from build123d import *

# Parameters (mm, degrees)
SKETCH_1_R      = 18
SKETCH_1_R_2    = 12
SKETCH_1_R_3    = 1.25
EXTRUDE_1_DEPTH = 5
EXTRUDE_START   = -2
SKETCH_2_R      = 12
SKETCH_2_R_2    = 10
EXTRUDE_2_DEPTH = 2
FILLET_1_R      = 1


with BuildPart() as part:
    # 草图1 → 凸台-拉伸1 (new body)
    with BuildSketch(Plane.XY):
        Circle(SKETCH_1_R)
        Circle(SKETCH_1_R_2, mode=Mode.SUBTRACT)
        with Locations((0, 15)):
            Circle(SKETCH_1_R_3, mode=Mode.SUBTRACT)
        with Locations((-15, 0)):
            Circle(SKETCH_1_R_3, mode=Mode.SUBTRACT)
        with Locations((0, -15)):
            Circle(SKETCH_1_R_3, mode=Mode.SUBTRACT)
        with Locations((15, 0)):
            Circle(SKETCH_1_R_3, mode=Mode.SUBTRACT)
    extrude(amount=EXTRUDE_1_DEPTH)

    # 草图2 → 凸台-拉伸2 (add)
    with BuildSketch(Plane.XY.offset(5).offset(EXTRUDE_START)):
        Circle(SKETCH_2_R)
        Circle(SKETCH_2_R_2, mode=Mode.SUBTRACT)
    extrude(amount=EXTRUDE_2_DEPTH)

    # 圆角1
    fillet_1_edges = [part.edges().sort_by_distance(p)[0] for p in [
        (-18, 0, 5),
    ]]
    fillet(fillet_1_edges, radius=FILLET_1_R)


solid = part.part
Geometry check sheet. Reference: the model listing, model coordinates, mm. A direction names the side the tool comes from. Round coordinates to 2 decimals unless told otherwise and drop trailing zeros. Order: outer loops, then holes, each group sorted by start corner. A loop starts at its lowest first (then second) coordinate and runs counter-clockwise, first axis right, second up. Notation, with made-up numbers: M -15.5,18.5 L 30.5,18.5 A18 ccw 30.5,42.5 Z; hole C -30,-35 d9. An arc over 180 degrees is marked long. Answer in a Markdown table with one row per item. Add a question column.
Item 1: Draft check along X on faces 1 (the face through (-12.3, 0.3, 0)), 2 (the face through (-0.16, -13.76, 2.46)), 3 (the face through (-2.343, 17.847, 1.972)), 4 (the face through (-11.99, 0.53, 1.48)). Enter one of: released by +X, released by -X, zero draft, split by the parting line, or undercut.
Item 2: Sectioned sample at B-B, the plane z = 1.55. Enter the section's corners in (x, y).
Item 3: Sectioned sample at C-C, the plane y = 0.5. State how many separate pieces and enclosed holes the cut face has, plus the area to 3 significant figures.
Item 4: Material ranges on L1, parallel to Y at x = 0, z = 2.4; L2, parallel to Y at x = 0, z = 4.6; L3, parallel to X at y = 7.5, z = 3.5, recorded low to high. Write a range as [from, to].
Item 5: Sectioned sample at A-A, the plane x = 0. Enter the section's corners in (y, z), plus the area to 3 significant figures.
Item 6: Set-up check for faces 5 (the face through (-5, 9, 3)), 6 (the face through (-2.17, -9.76, 3.99)): record each of +Z, -Z, +X, -X, +Y, -Y from which the full face is reachable in a straight line by a thin tool's end or side.
Item 7: Depth check by flat-ended pin: pin 1 Ø3 at (x, z) = (-5, 0.5) entering from +Y; pin 2 Ø10 at (x, y) = (6.5, 1.5) entering from -Z; pin 3 Ø3 at (x, z) = (-4, 0.5) entering from -Y. Enter the tip coordinate at first touch or a pass-through.
Filled in:
| question | item | result |
|---|---|---|
| 1 | face 1 | zero draft |
| 1 | face 2 | undercut |
| 1 | face 3 | split by the parting line |
| 1 | face 4 | undercut |
| 2 | outline | C 0,0 d36; hole C -15,0 d2.5; hole C 0,0 d24; hole C 0,-15 d2.5; hole C 0,15 d2.5; hole C 15,0 d2.5 |
| 3 | separate pieces | 4 |
| 3 | enclosed holes | 0 |
| 3 | area | 44.7 mm² |
| 4 | L1 | y = [-18, -16.25], [-13.75, -12], [12, 13.75], [16.25, 18] |
| 4 | L2 | y = [-17.8, -16.25], [-13.75, -10], [10, 13.75], [16.25, 17.8] |
| 4 | L3 | x = [-16.36, -6.61], [6.61, 16.36] |
| 5 | outline | M -18,0 L -16.25,0 L -16.25,5 L -17,5 A1 ccw -18,4 Z; M -13.75,0 L -12,0 L -12,3 L -10,3 L -10,5 L -13.75,5 Z; M 10,3 L 12,3 L 12,0 L 13.75,0 L 13.75,5 L 10,5 Z; M 16.25,0 L 18,0 L 18,4 A1 ccw 17,5 L 16.25,5 Z |
| 5 | area | 42.6 mm² |
| 6 | face 5 | -Z |
| 6 | face 6 | +Z, -Z |
| 7 | pin 1 | stops at y = 17.66 |
| 7 | pin 2 | stops at z = 3 |
| 7 | pin 3 | stops at y = -17.83 |
